Autodesk Inventor part; units mm, degrees
ref_plane "YZ Plane" through (0, 0, 0) normal (1, 0, 0) x (0, 1, 0)
ref_plane "XZ Plane" through (0, 0, 0) normal (0, 1, 0) x (-1, 0, 0)
ref_plane "XY Plane" through (0, 0, 0) normal (0, 0, 1) x (1, 0, 0)
sketch "Sketch1" plane through (0, 0, 0) normal (1, 0, 0) x (0, 1, 0)
  line L0 (0, 0) -> (155, 0)
  line L1 (155, 0) -> (155, -255)
  line L2 (155, -255) -> (0, -255)
  line L3 (0, -255) -> (0, 0)
  dimension "d1" = 255
  dimension "d2" = 155
extrude "Extrusion1" add sketch "Sketch1" against normal blind 320
sketch "Sketch2" plane through (0, 0, 0) normal (1, 0, 0) x (0, 0, -1)
  line L0 (0, 0) -> (0, 155)
  line L1 (255, 155) -> (255, 0)
  line L2 (0, 155) -> (255, 155)
  line L3 (255, 155) -> (255, 99.4837)
  line L4 (255, 99.4837) -> (0, 99.4837)
  line L5 (0, 99.4837) -> (0, 155)
  line L6 (30, 140) -> (225, 140)
  line L7 (225, 140) -> (225, 104.4837)
  line L8 (225, 104.4837) -> (30, 104.4837)
  line L9 (30, 104.4837) -> (30, 140)
  dimension "d8" = 15
  dimension "d9" = 5
  dimension "d10" = 30
  dimension "d11" = 30
extrude "Extrusion2" add sketch "Sketch2" along normal blind 3 contours L0 L2 L1 L4 | L6 L7 L8 L9
fillet "Fillet1" radius 2 4 edges at (3, 155, -127.5) (3, 127.2418, 0) (3, 127.2418, -255) (3, 99.4837, -127.5)
extrude "Extrusion3" cut sketch "Sketch2" along normal blind 3 and the other way blind 5 contours L6 L7 L8 L9
chamfer "Chamfer2" distance 18 distance2 6 1 edges at (3, 122.2418, -30) measured on face at (3, 148.6667, -95)
chamfer "Chamfer3" distance 18 distance2 6 1 edges at (3, 122.2418, -225) measured on face at (3, 148.6667, -95)
sketch "Sketch3" plane through (0, 0, 0) normal (1, 0, 0) x (0, 0, -1)
  ellipse E0 centre (19.9684, 15.0609) end of major axis (26.6774, 15.0609) minor radius 4.7478
  circle A0 centre (40, 71.92) radius 12.5
  line L0 (0, 0) -> (0, 99.4837)
  dimension "d25" = 25
  dimension "d34" = 40
extrude "Extrusion4" add sketch "Sketch3" along normal blind 8 contours E0
fillet "Fillet2" radius 2 1 edges at (8, 15.0609, -13.2594)
extrude "Extrusion5" add sketch "Sketch3" along normal blind 9 draft -4 contours A0
pattern_linear "Rectangular Pattern1" count 4 spacing 60 along (0, 0, -1) of "Extrusion5"
fillet "Fillet3" radius 10 6 edges at (-160, 0, 0) (2.4142, 154.4142, -0.5858) (-159.5, 155, 0) (-160, 0, -255) (2.4142, 154.4142, -254.4142) (-159.5, 155, -255)
equation "\"d11\" = d10"
properties part number "labortap1"
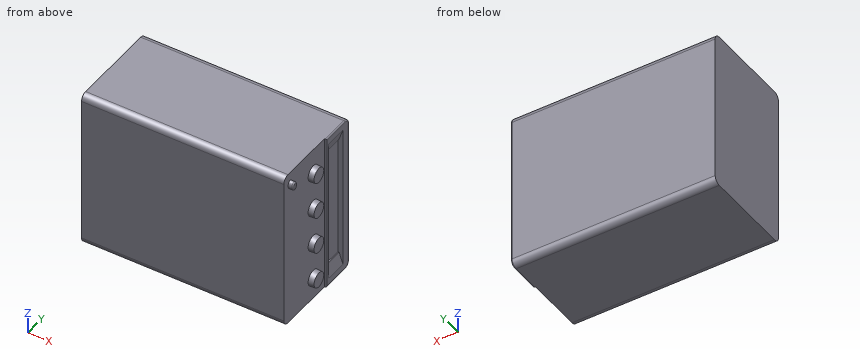
CAD build for the part. Positions are in the model's coordinates, mm. Give positions to 0.01 mm unless a question says otherwise; leave off trailing zeros. Order: outer loops, then holes, each group sorted by start corner. A loop starts at its lowest first (then second) coordinate and runs counter-clockwise, first axis right, second up. Notation, with made-up numbers: (31, 55.5) - (58, 55.5) arc R10 ccw to (58, 63.5) - close; hole circle Ø8 at (22, 57). An arc over 180 degrees is marked (long way). Answer in a Markdown table with one row per item.
1. Probe probe 1 along X at (y, z) = (69.5, -238.5); probe 2 along X at (y, z) = (143.5, -179.5); probe 3 along Z at (x, y) = (-13.5, 147). List the from-to ranges inside material, lowest first. Write a range as [from, to].
Data:
| item | result |
|---|---|
| probe 1 | x = [-320, 0] |
| probe 2 | x = [-320, 3] |
| probe 3 | z = [-254.8, -0.2] |
2. Saw through at B-B, the plane y = 123. Give the cut face in (x, z), plus the area to 3 significant figures.
Data:
| item | result |
|---|---|
| outline | (-320, -255) - (1, -255) arc R2 ccw to (3, -253) - (3, -243) - (-3, -225) - (-5, -225) - (-5, -30) - (-3, -30) - (3, -12) - (3, -2) arc R2 ccw to (1, 0) - (-320, 0) - close |
| area | 80,700 mm² |
3. Flat gauge pins, fed straight in: pin 1 (1 mm diameter, centred on y = 48.5, z = -74.5, fed in from +X); pin 2 (0.5 mm diameter, centred on x = 0.5, z = -177.5, fed in from -Y); pin 3 (18 mm diameter, centred on y = 125, z = -148, fed in from +X). Where does each tip first touch, or does it go through?
Data:
| item | result |
|---|---|
| pin 1 | stops at x = 0 |
| pin 2 | stops at y = 99.48 |
| pin 3 | stops at x = -5 |
4. Saw through at A-A, the plane z = -79. Give the cut face in (x, y), plus the area to 3 significant figures.
Data:
| item | result |
|---|---|
| outline | (-320, 0) - (0, 0) - (0, 99.48) - (1, 99.48) arc R2 ccw to (3, 101.48) - (3, 104.48) - (-5, 104.48) - (-5, 140) - (3, 140) - (3, 153) arc R2 ccw to (1, 155) - (-320, 155) - close |
| area | 49,500 mm² |
